from build123d import *

# Parameters (mm, degrees)
SKETCH1_W           = 55.8
SKETCH1_H           = 7
BOSS_EXTRUDE2_DEPTH = 6.3
SKETCH2_W           = 46.18
SKETCH2_H           = 2.31
CUT_EXTRUDE1_DEPTH  = 6.3
BOSS_EXTRUDE3_DEPTH = 6.3
SKETCH5_W           = 3
SKETCH5_H           = 24
BOSS_EXTRUDE4_DEPTH = 35.3
SKETCH6_R           = 2
SKETCH6_R_2         = 2.5
CUT_EXTRUDE2_DEPTH  = 40
BOSS_EXTRUDE5_DEPTH = 6.3
SKETCH8_W           = 3
SKETCH8_H           = 24
BOSS_EXTRUDE6_DEPTH = 2


with BuildPart() as part:
    # Sketch1 → Boss-Extrude2 (new body)
    with BuildSketch(Plane.XY):
        Rectangle(SKETCH1_W, SKETCH1_H)
    extrude(amount=BOSS_EXTRUDE2_DEPTH)

    # Sketch2 → Cut-Extrude1 (cut)
    with BuildSketch(Plane.XY.offset(6.3)):
        with Locations((1.51, 0.295)):
            Rectangle(SKETCH2_W, SKETCH2_H)
    extrude(amount=-CUT_EXTRUDE1_DEPTH, mode=Mode.SUBTRACT)

    # Sketch3 → Boss-Extrude3 (add)
    with BuildSketch(Plane.XY.offset(6.3)):
        Polygon((-23.42, 3.5), (-22.331, 6.494), (-21.209, 6.494), (-20.12, 3.5), align=None)
        Polygon((-19.26, 3.5), (-15.96, 3.5), (-17.049, 6.494), (-18.171, 6.494), align=None)
        Polygon((-15.1, 3.5), (-11.8, 3.5), (-12.889, 6.494), (-14.011, 6.494), align=None)
        Polygon((-10.94, 3.5), (-7.64, 3.5), (-8.729, 6.494), (-9.851, 6.494), align=None)
        Polygon((-6.78, 3.5), (-3.48, 3.5), (-4.569, 6.494), (-5.691, 6.494), align=None)
        Polygon((-2.62, 3.5), (0.68, 3.5), (-0.409, 6.494), (-1.531, 6.494), align=None)
        Polygon((1.54, 3.5), (4.84, 3.5), (3.751, 6.494), (2.629, 6.494), align=None)
        Polygon((5.7, 3.5), (9, 3.5), (7.911, 6.494), (6.789, 6.494), align=None)
        Polygon((9.86, 3.5), (13.16, 3.5), (12.071, 6.494), (10.949, 6.494), align=None)
        Polygon((14.02, 3.5), (17.32, 3.5), (16.231, 6.494), (15.109, 6.494), align=None)
        Polygon((18.18, 3.5), (21.48, 3.5), (20.391, 6.494), (19.269, 6.494), align=None)
        Polygon((22.34, 3.5), (25.64, 3.5), (24.551, 6.494), (23.429, 6.494), align=None)
    extrude(amount=-BOSS_EXTRUDE3_DEPTH)

    # Sketch5 → Boss-Extrude4 (add)
    with BuildSketch(Plane(origin=(0, -3.5, 0), x_dir=(-1, 0, 0), z_dir=(0, -1, 0))):
        with Locations((29.4, -3.15)):
            Rectangle(SKETCH5_W, SKETCH5_H)
    extrude(amount=-BOSS_EXTRUDE4_DEPTH)

    # Sketch6 → Cut-Extrude2 (cut)
    with BuildSketch(Plane(origin=(-27.9, 0, 0), x_dir=(0, 0, -1), z_dir=(1, 0, 0))):
        with Locations((4.35, -1.08)):
            Circle(SKETCH6_R)
        with Locations((-10.65, -1.08)):
            Circle(SKETCH6_R)
        with Locations((-3.15, 20.34)):
            Circle(SKETCH6_R_2)
    extrude(amount=-CUT_EXTRUDE2_DEPTH, mode=Mode.SUBTRACT)

    # Sketch7 → Boss-Extrude5 (add)
    with BuildSketch(Plane(origin=(0, 0, 0), x_dir=(-1, 0, 0), z_dir=(0, 0, -1))):
        Polygon((23.42, 3.5), (27.9, 16.274768446), (27.9, 8.809175652), (27.9, 3.5), align=None)
    extrude(amount=-BOSS_EXTRUDE5_DEPTH)

    # Sketch8 → Boss-Extrude6 (add)
    with BuildSketch(Plane.XZ.offset(3.5)):
        with Locations((-29.4, 3.15)):
            Rectangle(SKETCH8_W, SKETCH8_H)
    extrude(amount=BOSS_EXTRUDE6_DEPTH)


solid = part.part
Source: CAD feature listing. Evaluate the final solid. Frame: model axes, mm. A direction names the side the tool comes from. Round coordinates to 2 decimals unless told otherwise and drop trailing zeros. Loops run counter-clockwise (first coordinate to the right, second up) from the corner with the lowest first, then second, coordinate; pieces in that order, holes last. Notation, with made-up numbers: (-18.75, 1) - (18.25, 1) arc R29 ccw to (18.25, 40) - close; hole circle Ø2 at (78.25, 74). An arc over 180 degrees is marked (long way). Write item = value, one per line. Start each with the question number.
Item 1: Section query D-D on y = 11.5. Output: boundary loops of the cut face in (x, z), plus the area to 3 significant figures.
Item 2: Mould query, pull axis X, two halves, no side actions, for faces 4 (the face through (11.5, 6.494, 3.2)), 5 (the face through (25.1, 4.98, 3.19)), 6 (the face through (-12.34, 4.98, 3.19)). Classes: released by +X, released by -X, zero draft, split by the parting line, or undercut.
Item 3: Section query C-C on z = 3.15. Count the separate pieces of the cut face and the enclosed holes in it, plus the area to 3 significant figures.
Item 4: First-contact query: pin 1 Ø5 at (y, z) = (2, 11) entering from +X; pin 2 Ø0.6 at (x, z) = (15.5, 2.5) entering from +Y; pin 3 Ø6 at (x, z) = (5.5, 0.5) entering from -Y; pin 4 Ø3.5 at (y, z) = (-1.08, -4.35) entering from -X. Flat tips, straight axial feed; report the tip coordinate or a pass-through.
Item 5: Section query A-A on z = -4.35. Output: boundary loops of the cut face in (x, y), plus the area to 3 significant figures.
Item 6: Section query B-B on y = 20.34. Output: boundary loops of the cut face in (x, z).
Item 7: Reachability of faces 1 (the face through (24.6, 0, 3)), 2 (the face through (22.892, 5.018, 3.194)), 3 (the face through (24, 6.494, 3)) from +Z, -Z, +X, -X, +Y, -Y: full face, straight path, thin tool, end or side. Return the list, or none.
Item 8: Material intervals for line 1 (Y direction, x = -29.9, z = 10.65); line 2 (Z direction, x = -29, y = -1); line 3 (Y direction, x = -29.55, z = 3.15), sorted ascending.
Results list:
q1.outline = (-30.9, -8.85) - (-27.9, -8.85) - (-27.9, 0) - (-26.23, 0) - (-26.23, 6.3) - (-27.9, 6.3) - (-27.9, 15.15) - (-30.9, 15.15) - close
q1.area = 82.5 mm²
q2.face_4 = zero draft
q2.face_5 = released by +X
q2.face_6 = undercut
q3.separate_pieces = 2
q3.enclosed_holes = 1
q3.area = 489 mm²
q4.pin_1 = -27.9
q4.pin_2 = 6.49
q4.pin_3 = -3.5
q4.pin_4 = through
q5.outline = (-30.9, -5.5) - (-27.9, -5.5) - (-27.9, -3.08) - (-30.9, -3.08) - close; (-30.9, 0.92) - (-27.9, 0.92) - (-27.9, 31.8) - (-30.9, 31.8) - close
q5.area = 99.9 mm²
q6.outline = (-30.9, -8.85) - (-27.9, -8.85) - (-27.9, 0.65) - (-30.9, 0.65) - close; (-30.9, 5.65) - (-27.9, 5.65) - (-27.9, 15.15) - (-30.9, 15.15) - close
q7.face_1 = +Z, -Z
q7.face_2 = +Z, -Z, +Y
q7.face_3 = +Z, -Z, +X, +Y
q8.line_1 = -5.5 to -3.08, 0.92 to 31.8
q8.line_2 = -8.85 to -6.35, -2.35 to 8.65, 12.65 to 15.15
q8.line_3 = -5.5 to 17.84, 22.84 to 31.8
